from build123d import *

# Parameters (mm, degrees)
BASPROSKE_W         = 12
BASPROSKE_H         = 6.2139
TOOTHCUT_DEPTH      = 53.945557004
TEETHCUTS_COUNT     = 24
TEETHCUTS_ANGLE     = 345
BOSS_EXTRUDE1_START = -12
SKETCH1_R           = 46
SKETCH1_R_2         = 36.4385
BOSS_EXTRUDE1_DEPTH = 12
SKETCH2_R           = 2.5
CUT_EXTRUDE1_DEPTH  = 12


with BuildPart() as part:
    # BasProSke → Base-Revolve (revolve)
    with BuildSketch(Plane(origin=(0, 0, 0), x_dir=(1, 0, 0), z_dir=(0, 1, 0)), mode=Mode.PRIVATE) as base_revolve_sk:
        with Locations((6, 33.35695)):
            Rectangle(BASPROSKE_W, BASPROSKE_H)
    revolve(base_revolve_sk.sketch.rotate(Axis((-10, 0, 0), (1, 0, 0)), 180), axis=Axis((-10, 0, 0), (1, 0, 0)))

    # TooCutSke → ToothCut (cut, through all)
    with BuildSketch(Plane(origin=(0, 0, 0), x_dir=(0, 0, -1), z_dir=(1, 0, 0))):
        with BuildLine():
            ThreePointArc((3.32012603, 30.041691169), (2.184951712, 33.399149944), (0.358959887, 36.436731879))
            ThreePointArc((0.358959887, 36.436731879), (0, 36.4385), (-0.358959887, 36.436731879))
            ThreePointArc((-0.358959887, 36.436731879), (-2.184951712, 33.399149944), (-3.32012603, 30.041691169))
            ThreePointArc((-3.32012603, 30.041691169), (0, 30.2246), (3.32012603, 30.041691169))
        make_face()
    toothcut = extrude(amount=TOOTHCUT_DEPTH, mode=Mode.SUBTRACT)

    # TeethCuts: ToothCut ×24 about axis
    teethcuts_axis = Axis((-10, 0, 0), (1, 0, 0))
    for i in range(1, TEETHCUTS_COUNT):
        add(toothcut.rotate(teethcuts_axis, i * TEETHCUTS_ANGLE / (TEETHCUTS_COUNT - 1)), mode=Mode.SUBTRACT)

    # Sketch1 → Boss-Extrude1 (add)
    with BuildSketch(Plane(origin=(12, 0, 0), x_dir=(0, 0, -1), z_dir=(1, 0, 0)).offset(BOSS_EXTRUDE1_START)):
        Circle(SKETCH1_R)
        Circle(SKETCH1_R_2, mode=Mode.SUBTRACT)
    extrude(amount=BOSS_EXTRUDE1_DEPTH)

    # Sketch2 → Cut-Extrude1 (cut)
    with BuildSketch(Plane(origin=(12, 0, 0), x_dir=(0, 0, -1), z_dir=(1, 0, 0))):
        with Locations((41.25, 0)):
            Circle(SKETCH2_R)
        with Locations((0, -41.25)):
            Circle(SKETCH2_R)
        with Locations((-41.25, 0)):
            Circle(SKETCH2_R)
        with Locations((0, 41.25)):
            Circle(SKETCH2_R)
    extrude(amount=-CUT_EXTRUDE1_DEPTH, mode=Mode.SUBTRACT)


solid = part.part
Geometry: final body of the model. Coordinates: model frame, mm. Round coordinates to 2 decimals unless told otherwise and drop trailing zeros. Order: outer loops, then holes, each group sorted by start corner. A loop starts at its lowest first (then second) coordinate and runs counter-clockwise, first axis right, second up.
Q1. Section A-A, the plane z = -14.5. Output: boundary loops of the cut face in (x, y).
Result sheet:
outline: (0, -43.65) - (12, -43.65) - (12, -29.8) - (0, -29.8) - close; (0, 29.8) - (12, 29.8) - (12, 43.65) - (0, 43.65) - close
Q2. Section C-C, the plane x = 4.75. Give the number of separate pieces and of enclosed holes in the cut face, and give its area (3 significant figures).
Result sheet:
separate pieces: 1
enclosed holes: 5
area: 3,070 mm2
Q3. Pin query (flat end, axial travel): pin 1 (1.5 mm diameter, centred on x = 1.5, y = -29.5, fed in from -Z); pin 2 (1 mm diameter, centred on x = 2, y = -15, fed in from -Z); pin 3 (6 mm diameter, centred on x = 9, z = 1.5, fed in from -Y). Return the tip coordinate at first contact, or that it passes through.
Result sheet:
pin 1: stops at z = -35.91
pin 2: stops at z = -43.65
pin 3: stops at y = -46
Q4. Material intervals for probe 1 along Y at (x, z) = (8, 0); probe 2 along Z at (x, y) = (1.75, 31.5); probe 3 along Y at (x, z) = (2.75, -24), sorted ascending.
Result sheet:
probe 1: y = -46 to -43.75, -38.75 to -36.44, 36.44 to 38.75, 43.75 to 46
probe 2: z = -33.52 to -18.32, -17.38 to -10.79, -5.54 to -2.93, 2.93 to 5.54, 10.79 to 17.38, 18.32 to 33.52
probe 3: y = -39.24 to -25.74, -19.57 to -18.41, 18.41 to 19.57, 25.74 to 39.24
Q5. Section B-B, the plane y = 41.25. Output: boundary loops of the cut face in (x, z).
Result sheet:
outline: (0, -20.36) - (12, -20.36) - (12, -2.5) - (0, -2.5) - close; (0, 2.5) - (12, 2.5) - (12, 20.36) - (0, 20.36) - close
